Geometry check sheet. Reference: the model listing, model coordinates, mm. A direction names the side the tool comes from. Coordinates: 2 decimals unless noted, no trailing zeros. Loops run counter-clockwise (first coordinate to the right, second up) from the corner with the lowest first, then second, coordinate; pieces in that order, holes last. Notation, with made-up numbers: (-31, 4.25) - (-24, 4.25) arc R20 ccw to (-24, 11.25) - close; hole circle Ø9 at (41.25, 84.25). An arc over 180 degrees is marked (long way). One line per item, written item: value.
from build123d import *

# Parameters (mm, degrees)
BOSS_EXTRUDE1_DEPTH  = 10
SKETCH2_R            = 1.65
EXTERNAL_HOLES_DEPTH = 10
FILLET1_R            = 2
FILLET1_OF_MIRROR1_R = 2
SKETCH4_W            = 17
SKETCH4_H            = 1.5
BOSS_EXTRUDE2_DEPTH  = 14
SKETCH5_W            = 5.521728368
SKETCH5_H            = 8.571266928
BOSS_EXTRUDE3_DEPTH  = 10
CHAMFER1_SIZE        = 10


with BuildPart() as part:
    # Sketch1 → Boss-Extrude1 (new body)
    with BuildSketch(Plane.XY):
        with BuildLine():
            Line((-21, 0), (-11, 0))
            ThreePointArc((-11, 0), (-7.778174593, 7.778174593), (0, 11))
            Line((0, 11), (0, 16.170747429))
            Line((0, 16.170747429), (0, 25.35025486))
            Line((0, 25.35025486), (-12.324468849, 25.35025486))
            Line((-12.324468849, 25.35025486), (-16, 2.343730447))
            Line((-16, 2.343730447), (-21, 2.343730447))
            Line((-21, 2.343730447), (-21, 0))
        make_face()
    boss_extrude1 = extrude(amount=BOSS_EXTRUDE1_DEPTH)

    # Sketch2 → External_holes (cut)
    with BuildSketch(Plane(origin=(0, 2.343730447, 0), x_dir=(1, 0, 0), z_dir=(0, 1, 0))):
        with Locations(Location((-18.5, -5, 0), (0, 0, 180))):
            Circle(SKETCH2_R)
    external_holes = extrude(amount=-EXTERNAL_HOLES_DEPTH, mode=Mode.SUBTRACT)

    # Fillet1
    fillet1_edges = [part.edges().sort_by_distance(p)[0] for p in [
        (-21, 1.171865223, 10),
        (-21, 1.171865223, 0),
    ]]
    fillet(fillet1_edges, radius=FILLET1_R)

    # Mirror1: Boss-Extrude1, External_holes across Right Plane
    add(boss_extrude1.mirror(Plane(origin=(0, 0, 0), x_dir=(0, 0, -1), z_dir=(1, 0, 0))))
    add(external_holes.mirror(Plane(origin=(0, 0, 0), x_dir=(0, 0, -1), z_dir=(1, 0, 0))), mode=Mode.SUBTRACT)

    # Fillet1 of Mirror1
    fillet1_of_mirror1_edges = [part.edges().sort_by_distance(p)[0] for p in [
        (21, 1.171865223, 10),
        (21, 1.171865223, 0),
    ]]
    fillet(fillet1_of_mirror1_edges, radius=FILLET1_OF_MIRROR1_R)

    # Sketch4 → Boss-Extrude2 (add)
    with BuildSketch(Plane.XY.offset(10)):
        with Locations((0, 24.539717426)):
            Rectangle(SKETCH4_W, SKETCH4_H)
    extrude(amount=BOSS_EXTRUDE2_DEPTH)

    # Sketch5 → Boss-Extrude3 (add)
    with BuildSketch(Plane.XZ.offset(-23.789717426)):
        with Locations((0, 14.285633464)):
            Rectangle(SKETCH5_W, SKETCH5_H)
    extrude(amount=BOSS_EXTRUDE3_DEPTH)

    # Chamfer1
    # the kernel refuses this chamfer: 10 mm, written as the material it takes off along each edge
    with BuildSketch(Plane(origin=(-28.477694064, 13.789717426, 18.571266928), x_dir=(0, -0.027495876610586317, -0.9996219169112968), z_dir=(1, 0, 0))) as chamfer1_piece_1_section:
        Polygon((CHAMFER1_SIZE * 0.999621916911, CHAMFER1_SIZE * 0.0274958766106), (-CHAMFER1_SIZE * 0.0274958766106, CHAMFER1_SIZE * 0.999621916911), (0, 0), align=None)
    chamfer1_piece_1 = extrude(amount=56.955388128, mode=Mode.PRIVATE)
    chamfer1_piece_1 = split(chamfer1_piece_1, bisect_by=Plane(origin=(0, 17.174320664, 10), z_dir=(0, 0, 1)), keep=Keep.TOP, mode=Mode.PRIVATE)
    chamfer1_piece_1 = split(chamfer1_piece_1, bisect_by=Plane(origin=(0, 23.789717426, 15.454914499), z_dir=(0, -1, 0)), keep=Keep.TOP, mode=Mode.PRIVATE)
    add(chamfer1_piece_1, mode=Mode.SUBTRACT)


solid = part.part
(1) Material ranges on probe 1 along Z at (x, y) = (-18.5, 1.6); probe 2 along X at (y, z) = (1.5, 5.25); probe 3 along Z at (x, y) = (-9, 22.5), recorded low to high. Write a range as from..to.
Reply:
probe 1: 0..3.35, 6.65..10
probe 2: -21..-20.13, -16.87..-10.9, 10.9..16.87, 20.13..21
probe 3: 0..10
(2) Go/stop test with flat-tipped pins: pin 1 Ø1.6 at (y, z) = (24.5, 14) entering from +X; pin 2 Ø6 at (x, y) = (10.5, 15.5) entering from +Z; pin 3 Ø0.8 at (y, z) = (24.5, 19) entering from -X. Record where each tip stops, or that it passes through.
Reply:
pin 1: x = 8.5
pin 2: z = 10
pin 3: x = -8.5
(3) Cross-section at A-A on z = 5. Record the cut outline in (x, y), and give its area (3 significant figures).
Reply:
outline: (-21, 0) - (-20.15, 0) - (-20.15, 2.34) - (-21, 2.34) - close; (-16.85, 0) - (-11, 0) arc R11 cw to (11, 0) - (16.85, 0) - (16.85, 2.34) - (16, 2.34) - (12.32, 25.35) - (-12.32, 25.35) - (-16, 2.34) - (-16.85, 2.34) - close; (20.15, 0) - (21, 0) - (21, 2.34) - (20.15, 2.34) - close
area: 545 mm2
(4) Cross-section at C-C on y = 10. Record the cut outline in (x, z).
Reply:
outline: (-14.78, 0) - (-4.58, 0) - (-4.58, 10) - (-14.78, 10) - close; (4.58, 0) - (14.78, 0) - (14.78, 10) - (4.58, 10) - close
(5) Access from +Z, -Z, +X, -X, +Y, -Y to the whole of each face (thin tool, end or side, straight path). Record for faces 1 (the face through (-17, 2.344, 4)), 2 (the face through (2.761, 21, 13)), 3 (the face through (0, 23.79, 20)), 4 (the face through (-2.761, 21, 13)), 5 (the face through (8.5, 25, 17)).
Reply:
face 1: +Z, -Z, -X, +Y
face 2: +Z, +X, -Y
face 3: +Z, -Y
face 4: +Z, -X, -Y
face 5: +Z, +X, +Y, -Y
(6) Release check for a two-part mould opening along X. For faces 6 (the face through (17.19, 1.19, 4)), 7 (the face through (0, 13, 10)), 8 (the face through (-14.137, 14.008, 4.93)) record: pulls with the +X half, pulls with the -X half, needs draft (parallel to the pull), parting line crosses it, or undercut.
Reply:
face 6: undercut
face 7: needs draft
face 8: pulls with the -X half
(7) Cross-section at D-D on z = 9.25. Record the cut outline in (x, y).
Reply:
outline: (-20.56, 0) - (-11, 0) arc R11 cw to (11, 0) - (20.56, 0) - (20.56, 2.34) - (16, 2.34) - (12.32, 25.35) - (-12.32, 25.35) - (-16, 2.34) - (-20.56, 2.34) - close
(8) Cross-section at B-B on x = -18.5. Record the cut outline in (y, z), and give its area (3 significant figures).
Reply:
outline: (0, 0) - (2.34, 0) - (2.34, 3.35) - (0, 3.35) - close; (0, 6.65) - (2.34, 6.65) - (2.34, 10) - (0, 10) - close
area: 15.7 mm2
